from build123d import *

# Parameters (mm, degrees)
F1_DEPTH = 15
F2_R     = 2.5
F3_DEPTH = 0.5
F4_R     = 2


with BuildPart() as f1:
    # F0 (on Right) → F1 (new body, symmetric)
    with BuildSketch(Plane.YZ):
        Polygon((0, 0), (0, 14), (-60, 2), (-60, 0), align=None)
    extrude(amount=F1_DEPTH, both=True)

    # F2 (on face) → F3 (cut)
    with BuildSketch(Plane(origin=(0, 0, 0), x_dir=(1, 0, 0), z_dir=(0, 0, -1))):
        with Locations((0, 52)):
            Circle(F2_R)
        with Locations((10, 7)):
            Circle(F2_R)
        with Locations((-10, 7)):
            Circle(F2_R)
    extrude(amount=-F3_DEPTH, mode=Mode.SUBTRACT)

    # F4
    f4_edges = [f1.edges().sort_by_distance(p)[0] for p in [
        (15, -30, 8),
        (-15, -30, 8),
        (-15, 0, 7),
        (0, 0, 14),
        (15, 0, 7),
        (-15, -60, 1),
        (15, -60, 1),
    ]]
    fillet(f4_edges, radius=F4_R)


solid = f1.part
Source: CAD feature listing. Evaluate the final solid. Frame: model axes, mm. A direction names the side the tool comes from. Give positions to 0.01 mm unless a question says otherwise; leave off trailing zeros. Order: outer loops, then holes, each group sorted by start corner. A loop starts at its lowest first (then second) coordinate and runs counter-clockwise, first axis right, second up. Notation, with made-up numbers: (61, 26) -> (96, 26) arc R23 ccw to (96, 36) -> close; hole circle Ø9 at (-26.75, 84). An arc over 180 degrees is marked (long way). Use a Markdown table: item, result.
1) Mould query, pull axis Y, two halves, no side actions, for faces 3 (the cylindrical face through (14.2, -59.6, 0.8)), 4 (the flat face through (15, -24, 3)), 5 (the cylindrical face through (9.46, -4.56, 0.25)). Classes: +Y half, -Y half, draft (parallel to the pull), parting line (faces both ways), or undercut.
Answer list:
| item | result |
|---|---|
| face 3 | -Y half |
| face 4 | draft |
| face 5 | undercut |
2) Reachability of faces 1 (the flat face through (0.18, -30.79, 7.84)), 2 (the cylindrical face through (-12, -5.5, 0.2)) from +Z, -Z, +X, -X, +Y, -Y: full face, straight path, thin tool, end or side. Return the list, or none.
Answer list:
| item | result |
|---|---|
| face 1 | +Z, +X, -X, -Y |
| face 2 | -Z |
3) Contact query for flat-ended pins moving along their axis: P1, Ø8, axis at x = 10, y = -7, coming from the +Z side; P2, Ø2, axis at x = -2, y = -42.5, coming from the +Z side; P3, Ø6, axis at x = 7.5, y = -17, coming from the +Z side. Output: stop coordinate, or through.
Answer list:
| item | result |
|---|---|
| P1 | z = 13.4 |
| P2 | z = 5.7 |
| P3 | z = 11.2 |
4) Ray query, line 1 along X through (y, z) = (-7, 0.25); line 2 along Y through (x, z) = (-10, 0.3); line 3 along X through (y, z) = (-52, 0.45). Return the intervals inside material, ascending. Write a range as [from, to].
Answer list:
| item | result |
|---|---|
| line 1 | [-15, -12.5], [-7.5, 7.5], [12.5, 15] |
| line 2 | [-60, -9.5], [-4.5, 0] |
| line 3 | [-15, -2.5], [2.5, 15] |
5) Section query C-C, the plane x = 11. Return the cut outline in (y, z).
Answer list:
| item | result |
|---|---|
| outline | (-60, 0) -> (-9.29, 0) -> (-9.29, 0.5) -> (-4.71, 0.5) -> (-4.71, 0) -> (0, 0) -> (0, 11.56) arc R2 ccw to (-2.39, 13.52) -> (-60, 2) -> close |
6) Section query A-A, the plane x = 0. Return the cut outline in (y, z), then the cut area to 3 significant figures.
Answer list:
| item | result |
|---|---|
| outline | (-60, 0) -> (-54.5, 0) -> (-54.5, 0.5) -> (-49.5, 0.5) -> (-49.5, 0) -> (0, 0) -> (0, 11.56) arc R2 ccw to (-2.39, 13.52) -> (-60, 2) -> close |
| area | 476 mm² |
7) Section query B-B, the plane x = 6. Return the cut outline in (y, z), then the cut area to 3 significant figures.
Answer list:
| item | result |
|---|---|
| outline | (-60, 0) -> (0, 0) -> (0, 11.56) arc R2 ccw to (-2.39, 13.52) -> (-60, 2) -> close |
| area | 479 mm² |
